Could you check a few things on this model? Use its own coordinates, in mm. A direction names the side the tool comes from. Round coordinates to 2 decimals unless told otherwise and drop trailing zeros. Write each loop counter-clockwise with the first axis right and the second up, starting at its lowest first coordinate (ties: lowest second). Pieces come first, ordered by that corner, then holes. Notation, with made-up numbers: M 67,19 L 79,19 A13 ccw 79,31 Z; hole C 86,17.5 d4. An arc over 180 degrees is marked long. One line per item, written item: value. Start each with the question number.
(1) I want a section at C-C on y = 211.5. Please give me the cut outline in (x, z), and give its area (3 significant figures).
(2) If I drill on L1, parallel to Y at x = 0.3, z = 31; L2, parallel to Z at x = -0.45, y = 195.5; L3, parallel to Y at x = -0.8, z = 41, over which ranges is the centre line in solid material (lowest first)?
(3) Which directions (+Z, -Z, +X, -X, +Y, -Y) give clear straight access to the entire face, cutting with the end or side of a thin tool? Please do faces 5 (the face through (1.5, 203, 45)), 6 (the face through (-0.02, 234.15, 40.49)).
(4) I want a section at B-B on x = -0.35. Please give me the cut outline in (y, z), and give its area (3 significant figures).
(5) I want a section at A-A on z = 31. Please give me the cut outline in (x, y), and give its area (3 significant figures).
(6) Thinking about a two-plate mould opening in Y: for faces 1 (the face through (-0.02, 164.51, 40.65)), 2 (the face through (0, 237, -2)), 3 (the face through (0, 246.9, 9)), 4 (the face through (0, 242, -36.5)), which applies, released by +Y, released by -Y, zero draft, split by the parting line, or undercut?
(7) I want a section at D-D on z = 42. Please give me the cut outline in (x, y).
```python
from build123d import *

# Parameters (mm, degrees)
EXTRUDE_1_DEPTH = 3


with BuildPart() as part:
    # Эскиз1 → Бобышка-Вытянуть1 (new body)
    with BuildSketch(Plane(origin=(-1.5, 0, 0), x_dir=(0, -1, 0), z_dir=(-1, 0, 0))):
        with BuildLine():
            Line((-237, -36.5), (-237, 33.5))
            ThreePointArc((-237, 33.5), (-234.071067812, 40.571067812), (-227, 43.5))
            Line((-227, 43.5), (-171.5, 43.5))
            ThreePointArc((-171.5, 43.5), (-164.428932188, 40.571067812), (-161.5, 33.5))
            Line((-161.5, 33.5), (-161.5, -36.5))
            Line((-161.5, -36.5), (-151.6, -36.5))
            Line((-151.6, -36.5), (-151.6, 53.4))
            Line((-151.6, 53.4), (-246.9, 53.4))
            Line((-246.9, 53.4), (-246.9, -36.5))
            Line((-246.9, -36.5), (-237, -36.5))
        make_face()
    extrude(amount=-EXTRUDE_1_DEPTH)


solid = part.part
```
Found:
1. outline: M -1.5,43.5 L 1.5,43.5 L 1.5,53.4 L -1.5,53.4 Z
1. area: 29.7 mm²
2. L1: y = 151.6 to 161.5, 237 to 246.9
2. L2: z = 43.5 to 53.4
2. L3: y = 151.6 to 164.89, 233.61 to 246.9
3. face 5: +Z, -Z, +X, +Y, -Y
3. face 6: -Z, +X, -X
4. outline: M 151.6,-36.5 L 161.5,-36.5 L 161.5,33.5 A10 cw 171.5,43.5 L 227,43.5 A10 cw 237,33.5 L 237,-36.5 L 246.9,-36.5 L 246.9,53.4 L 151.6,53.4 Z
4. area: 2,570 mm²
5. outline: M -1.5,151.6 L 1.5,151.6 L 1.5,161.5 L -1.5,161.5 Z; M -1.5,237 L 1.5,237 L 1.5,246.9 L -1.5,246.9 Z
5. area: 59.4 mm²
6. face 1: undercut
6. face 2: undercut
6. face 3: released by +Y
6. face 4: zero draft
7. outline: M -1.5,151.6 L 1.5,151.6 L 1.5,166.23 L -1.5,166.23 Z; M -1.5,232.27 L 1.5,232.27 L 1.5,246.9 L -1.5,246.9 Z
